from build123d import *

# Parameters (mm, degrees)
F1_DEPTH = 2
F2_W     = 21.4
F2_H     = 3
F3_DEPTH = 10
F4_R     = 2
F5_R     = 2.3
F6_DEPTH = 25
F7_W     = 2.5
F7_H     = 8
F8_DEPTH = 25


with BuildPart() as f1:
    # F0 (on Top) → F1 (new body)
    with BuildSketch(Plane.XY):
        with BuildLine():
            Line((65.45691, 19.981824), (-66.14309, 19.981824))
            ThreePointArc((-66.14309, 19.981824), (-67.557303, 19.396037), (-68.14309, 17.981824))
            Line((-68.14309, 17.981824), (-68.14309, 9.181824))
            ThreePointArc((-68.14309, 9.181824), (-67.557303, 7.76761), (-66.14309, 7.181824))
            Line((-66.14309, 7.181824), (65.45691, 7.181824))
            ThreePointArc((65.45691, 7.181824), (66.871124, 7.76761), (67.45691, 9.181824))
            Line((67.45691, 9.181824), (67.45691, 17.981824))
            ThreePointArc((67.45691, 17.981824), (66.871124, 19.396037), (65.45691, 19.981824))
        make_face()
    extrude(amount=F1_DEPTH)

    # F2 (on face) → F3 (join)
    with BuildSketch(Plane.XY.offset(2)):
        with Locations((-55.34309, 10.681824)):
            Rectangle(F2_W, F2_H)
        with Locations((-55.34309, 16.481824)):
            Rectangle(F2_W, F2_H)
        with Locations((54.65691, 16.481824)):
            Rectangle(F2_W, F2_H)
        with Locations((54.65691, 10.681824)):
            Rectangle(F2_W, F2_H)
    extrude(amount=F3_DEPTH)

    # F4
    f4_edges = [f1.edges().sort_by_distance(p)[0] for p in [
        (-66.04309, 16.481824, 12),
        (-66.04309, 10.681824, 12),
        (-44.64309, 16.481824, 12),
        (-44.64309, 10.681824, 12),
        (43.95691, 16.481824, 12),
        (65.35691, 16.481824, 12),
        (65.35691, 10.681824, 12),
        (43.95691, 10.681824, 12),
    ]]
    fillet(f4_edges, radius=F4_R)

    # F5 (on face) → F6 (cut)
    with BuildSketch(Plane.XZ.offset(-9.181824)):
        with Locations((-55.34309, 8)):
            Circle(F5_R)
        with Locations((54.65691, 8)):
            Circle(F5_R)
    extrude(amount=-F6_DEPTH, mode=Mode.SUBTRACT)

    # F7 (on face) → F8 (cut)
    with BuildSketch(Plane(origin=(0, 0, 0), x_dir=(1, 0, 0), z_dir=(0, 0, -1))):
        Polygon((-37.84309, -9.181824), (-40.34309, -9.181824), (-40.34309, -17.181824), (-37.84309, -17.181824), (-37.84309, -12.181824), (-34.868522, -14.671218), (-31.893954, -12.181824), (-31.893954, -17.181824), (-29.393954, -17.181824), (-29.393954, -9.181824), (-31.893954, -9.181824), (-34.868522, -11.671218), align=None)
        Polygon((-25.244718, -9.181824), (-28.279638, -17.181824), (-25.779638, -17.181824), (-23.994718, -11.681824), (-22.25427, -17.181824), (-19.75427, -17.181824), (-22.744718, -9.181824), align=None)
        Polygon((-24.308708, -14.431824), (-24.887178, -16.214306), (-23.124494, -16.214306), (-23.688552, -14.431824), align=None)
        with BuildLine():
            ThreePointArc((-15.24951, -9.181824), (-17.37083, -10.060503), (-18.24951, -12.181824))
            Line((-18.24951, -12.181824), (-18.24951, -14.181824))
            ThreePointArc((-18.24951, -14.181824), (-17.37083, -16.303144), (-15.24951, -17.181824))
            Line((-15.24951, -17.181824), (-14.500879, -17.181824))
            ThreePointArc((-14.500879, -17.181824), (-13.139405, -16.855097), (-12.074485, -15.946083))
            Line((-12.074485, -15.946083), (-13.611591, -14.666511))
            ThreePointArc((-13.611591, -14.666511), (-14.240961, -15.06161), (-14.971134, -15.199663))
            ThreePointArc((-14.971134, -15.199663), (-15.814263, -15.003944), (-16.18885, -14.223651))
            Line((-16.18885, -14.223651), (-16.18885, -12.112802))
            ThreePointArc((-16.18885, -12.112802), (-15.814263, -11.332509), (-14.971134, -11.13679))
            ThreePointArc((-14.971134, -11.13679), (-14.240961, -11.274843), (-13.611591, -11.669942))
            Line((-13.611591, -11.669942), (-12.074485, -10.39037))
            ThreePointArc((-12.074485, -10.39037), (-13.134461, -9.500932), (-14.480871, -9.181824))
            Line((-14.480871, -9.181824), (-15.24951, -9.181824))
        make_face()
        Polygon((-7.34309, -9.181824), (-9.84309, -9.181824), (-9.84309, -17.181824), (-7.34309, -17.181824), (-7.34309, -14.431824), (-2.84309, -14.431824), (-2.84309, -17.181824), (-0.34309, -17.181824), (-0.34309, -9.181824), (-2.84309, -9.181824), (-2.84309, -11.931824), (-7.34309, -11.931824), align=None)
        with Locations((3.627188, -13.181824)):
            Rectangle(F7_W, F7_H)
        Polygon((10.021806, -9.181824), (7.521806, -9.181824), (7.521806, -17.181824), (10.021806, -17.181824), (10.021806, -12.771093), (14.303348, -17.181824), (16.803348, -17.181824), (16.803348, -9.181824), (14.303348, -9.181824), (14.303348, -13.592554), align=None)
        Polygon((20.67196, -9.181824), (17.637041, -17.181824), (20.137041, -17.181824), (21.92196, -11.681824), (23.662409, -17.181824), (26.162409, -17.181824), (23.17196, -9.181824), align=None)
        Polygon((21.0282, -16.214306), (22.792184, -16.214306), (22.228127, -14.431824), (21.60667, -14.431824), align=None)
        Polygon((33.219673, -12.990384), (29.436884, -17.181824), (32.436884, -17.181824), (34.647883, -14.731973), (36.65691, -17.181824), (39.65691, -17.181824), (36.219673, -12.990384), (39.65691, -9.181824), (36.65691, -9.181824), (34.791463, -11.248794), (33.09642, -9.181824), (30.09642, -9.181824), align=None)
    extrude(amount=-F8_DEPTH, mode=Mode.SUBTRACT)


solid = f1.part
The listing builds one solid part. Answer for the finished solid, in the listing's coordinates (mm). A direction names the side the tool comes from. Round coordinates to 2 decimals unless told otherwise and drop trailing zeros. Write each loop counter-clockwise with the first axis right and the second up, starting at its lowest first coordinate (ties: lowest second). Pieces come first, ordered by that corner, then holes. Notation, with made-up numbers: (3.25, 68) - (49.25, 68) arc R30 cw to (49.25, 95) - close; hole circle Ø6 at (-19, 53). An arc over 180 degrees is marked (long way). Use a Markdown table: item, result. Add a question column.
1. The part is cut by section B-B (x = 59.5). Write down the section's boundary in (y, z).
2. A tool of negligible diameter and unlimited length cuts with its end or side. For faces 1 (the face through (-55, 17.982, 5)), 2 (the face through (24.69, 13.24, 0.99)), 3 (the face through (-44.643, 11, 6)), 4 (the face through (-55, 9.182, 5)), from which of +Z, -Z, +X, -X, +Y, -Y can it reach the whole face along a straight path? Write none if from no direction.
3. For a pull along X with two mould halves and no side action, classify faces 5 (the face through (43.957, 11, 6)), 6 (the face through (65.357, 16, 6)), 7 (the face through (-55, 12.182, 5)) as +X half, -X half, draft (parallel to the pull), parting line (faces both ways), or undercut.
4. The part is cut by section C-C (x = 25). Write down the section's boundary in (y, z).
5. The part is cut by section A-A (z = 8). Give the number of separate pieces and of enclosed holes in the cut face, and give its area (3 significant figures).
6. Flat-ended cylindrical pins translate along their axes: P1, Ø0.9, axis at y = 16, z = 6.5, coming from the +X side; P2, Ø3.5, axis at y = 10, z = 4, coming from the -X side; P3, Ø1, axis at x = 12.5, y = 13, coming from the -Z side; P4, Ø2, axis at x = -13, y = 17, coming from the +Z side. Find the tip coordinate at first contact, or state that the pin passes through.
7. Consider line 1 (X direction, y = 16.75, z = 7.75); line 2 (Y direction, x = -62, z = 7.75); line 3 (X direction, y = 11.75, z = 3.25). Determine where each line is inside the solid, lowest interval first.
Reported:
| question | item | result |
|---|---|---|
| 1 | outline | (7.18, 0) - (19.98, 0) - (19.98, 2) - (17.98, 2) - (17.98, 12) - (14.98, 12) - (14.98, 2) - (12.18, 2) - (12.18, 12) - (9.18, 12) - (9.18, 2) - (7.18, 2) - close |
| 2 | face 1 | +Z, +X, -X, +Y |
| 2 | face 2 | +Z, -Z |
| 2 | face 3 | +Z, +Y, -Y |
| 2 | face 4 | +Z, +X, -X, -Y |
| 3 | face 5 | undercut |
| 3 | face 6 | +X half |
| 3 | face 7 | draft |
| 4 | outline | (7.18, 0) - (14.07, 0) - (14.07, 2) - (7.18, 2) - close; (17.18, 0) - (19.98, 0) - (19.98, 2) - (17.18, 2) - close |
| 5 | separate pieces | 8 |
| 5 | enclosed holes | 0 |
| 5 | area | 202 mm^2 |
| 6 | P1 | x = 65.36 |
| 6 | P2 | x = -66.04 |
| 6 | P3 | through |
| 6 | P4 | z = 2 |
| 7 | line 1 | -66.04 to -57.63, -53.06 to -44.64, 43.96 to 52.37, 56.94 to 65.36 |
| 7 | line 2 | 9.18 to 12.18, 14.98 to 17.98 |
| 7 | line 3 | -66.04 to -44.64, 43.96 to 65.36 |
